Input: part model. Units: mm. Frame: model coordinates. Face numbers are marked on the shaded views. Round coordinates to 2 decimals unless told otherwise and drop trailing zeros. Loops run counter-clockwise (first coordinate to the right, second up) from the corner with the lowest first, then second, coordinate; pieces in that order, holes last. Notation, with made-up numbers: (32.25, 19) -> (62.25, 19) arc R25 cw to (62.25, 46) -> close; hole circle Ø6 at (-3, 45.25). An arc over 180 degrees is marked (long way). Answer as a JSON object with one key per item and string values.
```python
from build123d import *

# Parameters (mm, degrees)
F0_W     = 30
F0_H     = 2
F1_DEPTH = 92.5
F2_W     = 30
F2_H     = 30
F3_DEPTH = 2
F4_W     = 30
F4_H     = 30
F5_DEPTH = 2
F6_R     = 3.175
F7_DEPTH = 250
F9_DEPTH = 25


with BuildPart() as f1:
    # F0 (on Right) → F1 (new body, symmetric)
    with BuildSketch(Plane.YZ):
        Rectangle(F0_W, F0_H)
    extrude(amount=F1_DEPTH, both=True)

    # F2 (on face) → F3 (join)
    with BuildSketch(Plane.YZ.offset(92.5)):
        with Locations((0, 16)):
            Rectangle(F2_W, F2_H)
    extrude(amount=-F3_DEPTH)

    # F4 (on face) → F5 (join)
    with BuildSketch(Plane(origin=(-92.5, 0, 0), x_dir=(0, -1, 0), z_dir=(-1, 0, 0))):
        with Locations((0, 16)):
            Rectangle(F4_W, F4_H)
    extrude(amount=-F5_DEPTH)

    # F6 (on face) → F7 (cut)
    with BuildSketch(Plane.YZ.offset(92.5)):
        with Locations((0, 15)):
            Circle(F6_R)
    extrude(amount=-F7_DEPTH, mode=Mode.SUBTRACT)

    # F8 (on face) → F9 (cut)
    with BuildSketch(Plane(origin=(0, 0, -1), x_dir=(1, 0, 0), z_dir=(0, 0, -1))):
        with BuildLine():
            ThreePointArc((30.5, -3.175), (32.7450640303, -2.2450640303), (33.675, 0))
            ThreePointArc((33.675, 0), (32.7450640303, 2.2450640303), (30.5, 3.175))
            ThreePointArc((30.5, 3.175), (27.325, 0), (30.5, -3.175))
        make_face()
        with BuildLine():
            ThreePointArc((30.5, -3.175), (27.325, 0), (30.5, 3.175))
            Line((30.5, 3.175), (-9.5, 3.175))
            ThreePointArc((-9.5, 3.175), (-7.2549359697, 2.2450640303), (-6.325, 0))
            ThreePointArc((-6.325, 0), (-7.2549359697, -2.2450640303), (-9.5, -3.175))
            Line((-9.5, -3.175), (30.5, -3.175))
        make_face()
        with BuildLine():
            ThreePointArc((-6.325, 0), (-7.2549359697, 2.2450640303), (-9.5, 3.175))
            ThreePointArc((-9.5, 3.175), (-12.675, 0), (-9.5, -3.175))
            ThreePointArc((-9.5, -3.175), (-7.2549359697, -2.2450640303), (-6.325, 0))
        make_face()
    extrude(amount=-F9_DEPTH, mode=Mode.SUBTRACT)


solid = f1.part
```
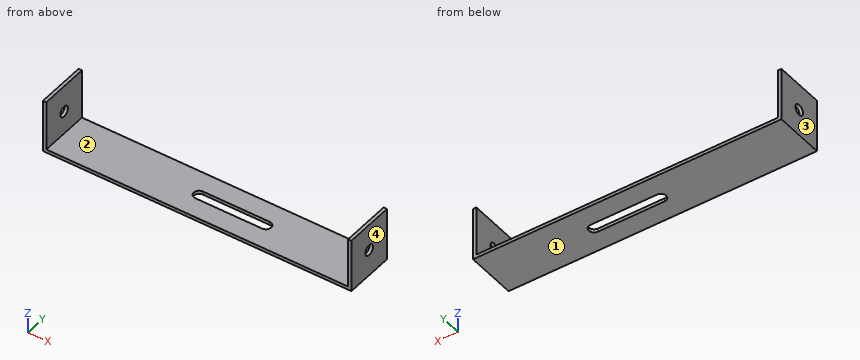
1) Section C-C, the plane z = 15. Output: boundary loops of the cut face in (x, y) (3 decimals), plus the area to 3 significant figures.
Output:
{"outline": "(-92.5, -15) -> (-90.5, -15) -> (-90.5, -3.175) -> (-92.5, -3.175) -> close; (-92.5, 3.175) -> (-90.5, 3.175) -> (-90.5, 15) -> (-92.5, 15) -> close; (90.5, -15) -> (92.5, -15) -> (92.5, -3.175) -> (90.5, -3.175) -> close; (90.5, 3.175) -> (92.5, 3.175) -> (92.5, 15) -> (90.5, 15) -> close", "area": "94.6 mm^2"}
2) Contact query for flat-ended pins moving along their axis: P1, Ø5, axis at y = 0, z = 15, coming from the +X side; P2, Ø6, axis at x = -49, y = 4.5, coming from the +Z side. Output: stop coordinate, or through.
Output:
{"P1": "passes through", "P2": "stops at z = 1"}
3) Draft query along X for the marked faces 1, 2, 3 and 4. Return one class per face: +X half, -X half, draft (parallel to the pull), parting line (faces both ways), or undercut.
Output:
{"face 1": "draft", "face 2": "undercut", "face 3": "-X half", "face 4": "+X half"}
4) Section D-D, the plane y = 8.5. Output: boundary loops of the cut face in (x, z).
Output:
{"outline": "(-92.5, -1) -> (92.5, -1) -> (92.5, 31) -> (90.5, 31) -> (90.5, 1) -> (-90.5, 1) -> (-90.5, 31) -> (-92.5, 31) -> close"}
5) Section B-B, the plane x = 19. Output: boundary loops of the cut face in (y, z) (3 decimals).
Output:
{"outline": "(-15, -1) -> (-3.175, -1) -> (-3.175, 1) -> (-15, 1) -> close; (3.175, -1) -> (15, -1) -> (15, 1) -> (3.175, 1) -> close"}
6) Section A-A, the plane z = 23. Output: boundary loops of the cut face in (x, y), plus the area to 3 significant figures.
Output:
{"outline": "(-92.5, -15) -> (-90.5, -15) -> (-90.5, 15) -> (-92.5, 15) -> close; (90.5, -15) -> (92.5, -15) -> (92.5, 15) -> (90.5, 15) -> close", "area": "120 mm^2"}
7) Ray query, probe 1 along X at (y, z) = (-9.25, 21); probe 2 along Z at (x, y) = (-91.2, 0) (3 decimals); probe 3 along Z at (x, y) = (-47.5, 0.75). Return the intervals inside material, ascending.
Output:
{"probe 1": "x = -92.5 to -90.5, 90.5 to 92.5", "probe 2": "z = -1 to 11.825, 18.175 to 31", "probe 3": "z = -1 to 1"}
